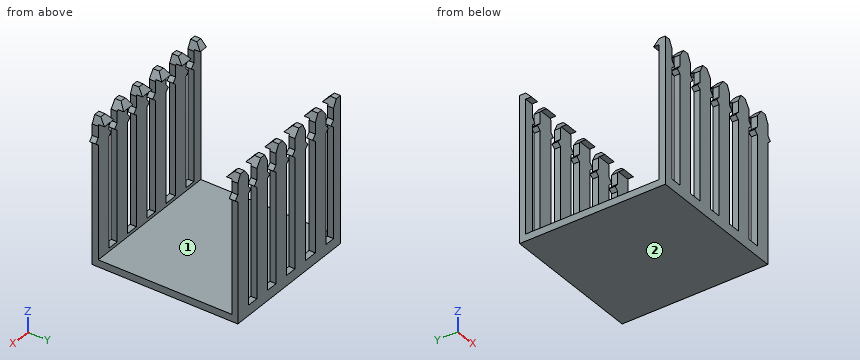
```python
from build123d import *

# Parameters (mm, degrees)
F1_DEPTH = 76.2
F3_DEPTH = 76.175829


with BuildPart() as f1:
    # F0 (on Front) → F1 (new body)
    with BuildSketch(Plane.XZ):
        Polygon((-35.158783, 38.1), (-38.1, 38.1), (-38.1, -32.752417), (-33.137847, -32.752417), (-33.137847, 24.566615), (-31.27237, 26.165593), (-33.137847, 28.341984), (-33.137847, 34.249332), align=None)
        Polygon((-33.137847, -32.752417), (-38.1, -32.752417), (-38.1, -38.1), (36.209352, -38.1), (36.209352, -32.752417), (28.591979, -32.752417), (22.460993, -32.752417), (14.84362, -32.752417), (8.592682, -32.752417), (0.975309, -32.752417), (-5.155675, -32.752417), (-12.773048, -32.752417), (-19.924045, -32.752417), (-27.541418, -32.752417), align=None)
        Polygon((-27.541418, 24.566615), (-27.541418, -32.752417), (-19.924045, -32.752417), (-19.924045, 24.566615), (-18.058568, 26.165593), (-19.924045, 28.341984), (-19.924045, 34.249332), (-21.789523, 38.1), (-24.743196, 38.1), (-27.541414, 34.249332), (-27.541414, 28.341984), (-29.406892, 26.165593), align=None)
        Polygon((28.591979, -32.752417), (36.209352, -32.752417), (36.209352, 24.566615), (38.074829, 26.165593), (36.209352, 28.341984), (36.209352, 34.249332), (34.343874, 38.1), (31.390201, 38.1), (28.591983, 34.249332), (28.591983, 28.341984), (26.726505, 26.165593), (28.591979, 24.566615), align=None)
        Polygon((-12.773048, 24.566615), (-12.773048, -32.752417), (-5.155675, -32.752417), (-5.155675, 24.566615), (-3.290201, 26.165593), (-5.155679, 28.341984), (-5.155679, 34.249332), (-7.953897, 38.1), (-10.90757, 38.1), (-12.773048, 34.249332), (-12.773048, 28.341984), (-14.638525, 26.165593), align=None)
        Polygon((14.84362, -32.752417), (22.460993, -32.752417), (22.460993, 24.566615), (24.326468, 26.165593), (22.46099, 28.341984), (22.46099, 34.249332), (19.662771, 38.1), (16.709099, 38.1), (14.84362, 34.249332), (14.84362, 28.341984), (12.978144, 26.165593), (14.84362, 24.566615), align=None)
        Polygon((0.975309, 24.566615), (0.975309, -32.752417), (8.592682, -32.752417), (8.592682, 24.566615), (10.458158, 26.165593), (8.592682, 28.341984), (8.592682, 34.249332), (6.727204, 38.1), (3.773531, 38.1), (0.975313, 34.249332), (0.975313, 28.341984), (-0.890166, 26.165593), align=None)
    extrude(amount=F1_DEPTH)

    # F2 (on face) → F3 (cut, through all)
    with BuildSketch(Plane(origin=(-38.1, 0, 0), x_dir=(0, -1, 0), z_dir=(-1, 0, 0))):
        Polygon((73.025, 38.1), (3.175, 38.1), (6.136249, 34.965612), (3.175, 34.965612), (3.175, -34.434266), (73.025, -34.434266), (73.025, 34.965612), (70.063751, 34.965612), align=None)
    extrude(amount=-F3_DEPTH, mode=Mode.SUBTRACT)


solid = f1.part
```
Check sheet for the modelled part. Datum: model origin and axes. Units: mm. Face numbers are marked on the shaded views. Round coordinates to 2 decimals unless told otherwise and drop trailing zeros. Loops run counter-clockwise (first coordinate to the right, second up) from the corner with the lowest first, then second, coordinate; pieces in that order, holes last. Notation, with made-up numbers: (47.5, 2) -> (92.5, 2) arc R13 cw to (92.5, 10) -> close; hole circle Ø9 at (81.5, 89). An arc over 180 degrees is marked (long way). Write item = value, one per line. Start each with the question number.
1) Release check for a two-part mould opening along Y. For the marked faces 1 and 2 record: released by +Y, released by -Y, zero draft, split by the parting line, or undercut.
2) Sectioned sample at A-A, the plane z = -29.5. State how many separate pieces and enclosed holes the cut face has, plus the area to 3 significant figures.
3) Gauge pin test, flat ends, axial feed: pin 1 Ø1.6 at (y, z) = (-1, 32) entering from +X; pin 2 Ø2.5 at (x, y) = (24.5, -2) entering from +Z; pin 3 Ø1.6 at (x, y) = (-0.5, -1.5) entering from +Z. Record the tip position at first contact, or that the pin passes through.
4) Sectioned sample at B-B, the plane y = -42. Record the cut outline in (x, z), plus the area to 3 significant figures.
5) Thickness scan on probe 1 along Y at (x, z) = (-22.5, 28) (3 decimals); probe 2 along Z at (x, y) = (26, -48); probe 3 along Z at (x, y) = (-6.5, -71). Record the ranges inside material, lowest first.
Results are:
q1.face_1 = undercut
q1.face_2 = zero draft
q2.separate_pieces = 12
q2.enclosed_holes = 0
q2.area = 273 mm^2
q3.pin_1 = 36.21
q3.pin_2 = 27.42
q3.pin_3 = 27.55
q4.outline = (-38.1, -38.1) -> (36.21, -38.1) -> (36.21, -34.43) -> (-38.1, -34.43) -> close
q4.area = 272 mm^2
q5.probe_1 = -76.2 to -73.025, -3.175 to 0
q5.probe_2 = -38.1 to -34.43
q5.probe_3 = -38.1 to -34.43, 34.97 to 35.96
